from build123d import *

# Parameters (mm, degrees)
SKETCH1_W                                 = 68.0085
SKETCH1_H                                 = 68.0085
SKETCH1_W_2                               = 60.0583
SKETCH1_H_2                               = 60.0583
BOSS_EXTRUDE1_DEPTH                       = 24.0665
F_7_16_0_4375_DIAMETER_HOLE1_D            = 11.1125
SKETCH10_W                                = 16.002
SKETCH10_H                                = 30.0482
BOSS_EXTRUDE2_DEPTH                       = 3.9751
FILLET1_R                                 = 6.35
FILLET1_OF_MIRROR1_R                      = 6.35
FILLET2_R                                 = 6.35
FILLET3_R                                 = 6.35
CSK_FOR_6_FLAT_HEAD_MACHINE_SCREW_2_COUNT = 2
CSK_FOR_6_FLAT_HEAD_MACHINE_SCREW_2_PITCH = 19.8882


with BuildPart() as part:
    # Sketch1 → Boss-Extrude1 (new body)
    with BuildSketch(Plane.XY):
        Rectangle(SKETCH1_W, SKETCH1_H)
        Rectangle(SKETCH1_W_2, SKETCH1_H_2, mode=Mode.SUBTRACT)
    extrude(amount=BOSS_EXTRUDE1_DEPTH)

    # 7/16 (0.4375) Diameter Hole1 (through all)
    with Locations(Plane(origin=(34.00425, 0, 0), x_dir=(0, 0, -1), z_dir=(1, 0, 0))):
        with Locations((-12.03325, 0)):
            Hole(F_7_16_0_4375_DIAMETER_HOLE1_D / 2)

    # Sketch10 → Boss-Extrude2 (add)
    with BuildSketch(Plane.ZY.offset(34.00425)):
        with Locations((32.0675, 0)):
            Rectangle(SKETCH10_W, SKETCH10_H)
    boss_extrude2 = extrude(amount=-BOSS_EXTRUDE2_DEPTH)

    # Fillet1
    fillet1_edges = [part.edges().sort_by_distance(p)[0] for p in [
        (-32.0167, -15.0241, 24.0665),
        (-32.0167, 15.0241, 24.0665),
    ]]
    fillet(fillet1_edges, radius=FILLET1_R)

    # Mirror1: Boss-Extrude2 across plane
    add(boss_extrude2.mirror(Plane(origin=(0, 0, 0), x_dir=(0, 0, 1), z_dir=(1, 0, 0))))

    # Fillet1 of Mirror1
    fillet1_of_mirror1_edges = [part.edges().sort_by_distance(p)[0] for p in [
        (32.0167, -15.0241, 24.0665),
        (32.0167, 15.0241, 24.0665),
    ]]
    fillet(fillet1_of_mirror1_edges, radius=FILLET1_OF_MIRROR1_R)

    # Fillet2
    fillet2_edges = [part.edges().sort_by_distance(p)[0] for p in [
        (34.00425, -34.00425, 12.03325),
        (-34.00425, -34.00425, 12.03325),
        (-34.00425, 34.00425, 12.03325),
        (34.00425, 34.00425, 12.03325),
    ]]
    fillet(fillet2_edges, radius=FILLET2_R)

    # Fillet3
    fillet3_edges = [part.edges().sort_by_distance(p)[0] for p in [
        (30.02915, -30.02915, 12.03325),
        (30.02915, 30.02915, 12.03325),
        (-30.02915, 30.02915, 12.03325),
        (-30.02915, -30.02915, 12.03325),
    ]]
    fillet(fillet3_edges, radius=FILLET3_R)

    # Sketch14 → CSK for #6 Flat Head Machine Screw (100)1 (revolve, cut)
    with BuildSketch(Plane(origin=(-34.00425, 9.9441, 36.2585), x_dir=(0, 0, 1), z_dir=(0, 1, 0))):
        Polygon((0, 0), (0, 10.538824014), (1.89865, 9.398), (1.89865, 1.380025208), (3.5433, 0), align=None)
    csk_for_6_flat_head_machine_screw_100 = revolve(axis=Axis((-40.35425, 9.9441, 36.2585), (1, 0, 0)), mode=Mode.SUBTRACT)

    # CSK for _6 Flat Head Machine Screw _ 2: CSK for #6 Flat Head Machine Screw (100)1 ×2
    with Locations(*[(0, -i * CSK_FOR_6_FLAT_HEAD_MACHINE_SCREW_2_PITCH, 0) for i in range(1, CSK_FOR_6_FLAT_HEAD_MACHINE_SCREW_2_COUNT)]):
        add(csk_for_6_flat_head_machine_screw_100, mode=Mode.SUBTRACT)

    # Mirror2: CSK for #6 Flat Head Machine Screw (100)1 across plane
    add(csk_for_6_flat_head_machine_screw_100.mirror(Plane(origin=(0, 0, 0), x_dir=(0, 0, 1), z_dir=(1, 0, 0))), mode=Mode.SUBTRACT)

    # Mirror2 copy 1 sketch → Mirror2 copy 1 (revolve, cut)
    with BuildSketch(Plane(origin=(34.00425, -9.9441, 36.2585), x_dir=(0, 0, 1), z_dir=(0, 1, 0))):
        Polygon((0, 0), (0, -10.538824014), (1.89865, -9.398), (1.89865, -1.380025208), (3.5433, 0), align=None)
    revolve(axis=Axis((40.35425, -9.9441, 36.2585), (1, 0, 0)), mode=Mode.SUBTRACT)


solid = part.part
Source: CAD feature listing. Evaluate the final solid. Frame: model axes, mm. A direction names the side the tool comes from. Give positions to 0.01 mm unless a question says otherwise; leave off trailing zeros. Order: outer loops, then holes, each group sorted by start corner. A loop starts at its lowest first (then second) coordinate and runs counter-clockwise, first axis right, second up. Notation, with made-up numbers: (-37, 31.5) -> (-32, 31.5) arc R30 cw to (-32, 59.5) -> close; hole circle Ø10 at (80, 19.5). An arc over 180 degrees is marked (long way). Write item = value, one per line.
Q1. Material intervals for line 1 (Y direction, x = 1, z = 19.5); line 2 (Z direction, x = -27, y = 30), sorted ascending. Write a range as from..to.
Data:
line_1 = -34..-30.03, 30.03..34
line_2 = 0..24.07
Q2. Cut plane B-B, the plane x = 1. Output: boundary loops of the cut face in (y, z), and give its area (3 significant figures).
Data:
outline = (-34, 0) -> (-30.03, 0) -> (-30.03, 24.07) -> (-34, 24.07) -> close; (30.03, 0) -> (34, 0) -> (34, 24.07) -> (30.03, 24.07) -> close
area = 191 mm^2
Q3. Pin query (flat end, axial travel): pin 1 (10 mm diameter, centred on y = 0, z = 12.03, fed in from +X); pin 2 (6 mm diameter, centred on y = 9.94, z = 36.26, fed in from -X); pin 3 (14 mm diameter, centred on x = 12.5, y = -29.5, fed in from +Z); pin 4 (4.5 mm diameter, centred on x = 32.5, z = 35.5, fed in from -Y). Return the tip coordinate at first contact, or that it passes through.
Data:
pin_1 = through
pin_2 = -33.55
pin_3 = 24.07
pin_4 = -15.02
Q4. Cut plane C-C, the plane z = 9. Output: boundary loops of the cut face in (x, y), and give its area (3 significant figures).
Data:
outline = (-34, -27.65) arc R6.35 ccw to (-27.65, -34) -> (27.65, -34) arc R6.35 ccw to (34, -27.65) -> (34, -4.66) -> (30.03, -4.66) -> (30.03, -23.68) arc R6.35 cw to (23.68, -30.03) -> (-23.68, -30.03) arc R6.35 cw to (-30.03, -23.68) -> (-30.03, -4.66) -> (-34, -4.66) -> close; (-34, 4.66) -> (-30.03, 4.66) -> (-30.03, 23.68) arc R6.35 cw to (-23.68, 30.03) -> (23.68, 30.03) arc R6.35 cw to (30.03, 23.68) -> (30.03, 4.66) -> (34, 4.66) -> (34, 27.65) arc R6.35 ccw to (27.65, 34) -> (-27.65, 34) arc R6.35 ccw to (-34, 27.65) -> close
area = 944 mm^2
Q5. Cut plane A-A, the plane y = 0. Output: boundary loops of the cut face in (x, z), and give its area (3 significant figures).
Data:
outline = (-34, 0) -> (-30.03, 0) -> (-30.03, 6.48) -> (-34, 6.48) -> close; (-34, 17.59) -> (-30.03, 17.59) -> (-30.03, 40.07) -> (-34, 40.07) -> close; (30.03, 0) -> (34, 0) -> (34, 6.48) -> (30.03, 6.48) -> close; (30.03, 17.59) -> (34, 17.59) -> (34, 40.07) -> (30.03, 40.07) -> close
area = 230 mm^2
Q6. Cut plane D-D, the plane y = -20.5. Output: boundary loops of the cut face in (x, z), and give its area (3 significant figures).
Data:
outline = (-34, 0) -> (-30.03, 0) -> (-30.03, 24.13) -> (-34, 24.13) -> close; (30.03, 0) -> (34, 0) -> (34, 24.13) -> (30.03, 24.13) -> close
area = 192 mm^2
Q7. Pull-direction query (Z, two-part tool) for faces 1 (the face through (32, -15.024, 35)), 2 (the face through (-32, 0, 40.068)), 3 (the face through (-31.34, -10.03, 34.36)), 4 (the face through (-32.045, 0.244, 6.482)); classes: released by +Z, released by -Z, zero draft, split by the parting line, or undercut.
Data:
face_1 = zero draft
face_2 = released by +Z
face_3 = undercut
face_4 = undercut
Q8. Set-up query: faces 5 (the face through (30.029, 0, 20)), 6 (the face through (-32, 15.024, 35)), 7 (the face through (0, -34.004, 12)). Return all of +Z, -Z, +X, -X, +Y, -Y with unobstructed straight access to the full face (end or side cutting, diameter ignored); none if empty.
Data:
face_5 = +Z, -Z
face_6 = +Z, +X, -X, +Y
face_7 = +Z, -Z, +X, -X, -Y
